```python
from build123d import *

# Parameters (mm, degrees)
F1_DEPTH = 30


with BuildPart() as f1:
    # F0 (on Front) → F1 (new body)
    with BuildSketch(Plane.XZ):
        Polygon((30, 50), (30, 0), (1135, 0), (1135, 50), (1170, 50), (1170, 150), (1135, 150), (1135, 200), (30, 200), (30, 150), (-5, 150), (-5, 50), align=None)
        with BuildLine():
            Line((312.5, 50), (112.5, 50))
            ThreePointArc((112.5, 50), (62.5, 100), (112.5, 150))
            Line((112.5, 150), (312.5, 150))
            ThreePointArc((312.5, 150), (362.5, 100), (312.5, 50))
        make_face(mode=Mode.SUBTRACT)
        with BuildLine():
            Line((682.5, 50), (482.5, 50))
            ThreePointArc((482.5, 50), (432.5, 100), (482.5, 150))
            Line((482.5, 150), (682.5, 150))
            ThreePointArc((682.5, 150), (732.5, 100), (682.5, 50))
        make_face(mode=Mode.SUBTRACT)
        with BuildLine():
            Line((1052.5, 50), (852.5, 50))
            ThreePointArc((852.5, 50), (802.5, 100), (852.5, 150))
            Line((852.5, 150), (1052.5, 150))
            ThreePointArc((1052.5, 150), (1102.5, 100), (1052.5, 50))
        make_face(mode=Mode.SUBTRACT)
    extrude(amount=F1_DEPTH)


solid = f1.part
```
The model under review builds one solid part; all positions refer to its coordinate system, in mm. A direction names the side the tool comes from. Coordinates: 2 decimals unless noted, no trailing zeros. Write each loop counter-clockwise with the first axis right and the second up, starting at its lowest first coordinate (ties: lowest second). Pieces come first, ordered by that corner, then holes. Notation, with made-up numbers: (20.5, 52) -> (51.5, 52) arc R22 ccw to (51.5, 69) -> close; hole circle Ø8 at (60.5, 86). An arc over 180 degrees is marked (long way). One line per item, written item: value. Start each with the question number.
Q1. Clearance check with flat-ended pins moving along their axes: P1, Ø9, axis at x = 1157.5, y = -20, coming from the -Z side; P2, Ø9, axis at y = -20.5, z = 168.5, coming from the -X side; P3, Ø15, axis at x = 5.5, y = -15, coming from the +Z side. State where each tip first meets the part, or that it passes through.
Q2. To check wall thickness, follow probe 1 along Z at (x, y) = (303, -5); probe 2 along X at (y, z) = (-16, 138); probe 3 along X at (y, z) = (-14, 54.5). State the ranges of each line that lie inside material, in increasing order.
Q3. The part is to be moulded in two halves that separate along X. For faces 1 (the face through (1135, -15, 175)), 2 (the face through (584, -15, 50)), 3 (the face through (-5, -15, 101)), say which applies: +X half, -X half, draft (parallel to the pull), parting line (faces both ways), or undercut.
Q4. Add section A-A, the plane x = 990. Give the boundary of the cut face in (y, z), then the cut area to 3 significant figures.
Q5. Add section C-C, the plane y = -20.75. Give the boundary of the cut face in (x, z), then the cut area to 3 significant figures.
Q6. For faces 4 (the face through (30, -15, 175)), 5 (the face through (30, -15, 25)), 6 (the face through (954, -15, 50)), list the 3-axis set-ups (+Z, -Z, +X, -X, +Y, -Y) from which the entire face can be reached by the end or side of a thin tool; tool diameter is ignored.
Q7. Add section B-B, the plane z = 100. Give the boundary of the cut face in (x, y), then the cut area to 3 significant figures.
Q8. Add section D-D, the plane z = 13. Give the boundary of the cut face in (x, y), then the cut area to 4 significant figures.
Response:
1. P1: z = 50
1. P2: x = 30
1. P3: z = 150
2. probe 1: 0 to 50, 150 to 200
2. probe 2: -5 to 80, 345 to 450, 715 to 820, 1085 to 1170
2. probe 3: -5 to 91.77, 333.23 to 461.77, 703.23 to 831.77, 1073.23 to 1170
3. face 1: +X half
3. face 2: undercut
3. face 3: -X half
4. outline: (-30, 0) -> (0, 0) -> (0, 50) -> (-30, 50) -> close; (-30, 150) -> (0, 150) -> (0, 200) -> (-30, 200) -> close
4. area: 3,000 mm²
5. outline: (-5, 50) -> (30, 50) -> (30, 0) -> (1135, 0) -> (1135, 50) -> (1170, 50) -> (1170, 150) -> (1135, 150) -> (1135, 200) -> (30, 200) -> (30, 150) -> (-5, 150) -> close; hole (112.5, 50) -> (312.5, 50) arc R50 ccw to (312.5, 150) -> (112.5, 150) arc R50 ccw to start; hole (482.5, 50) -> (682.5, 50) arc R50 ccw to (682.5, 150) -> (482.5, 150) arc R50 ccw to start; hole (852.5, 50) -> (1052.5, 50) arc R50 ccw to (1052.5, 150) -> (852.5, 150) arc R50 ccw to start
5. area: 144,000 mm²
6. face 4: +Z, -X, +Y, -Y
6. face 5: -Z, -X, +Y, -Y
6. face 6: +Y, -Y
7. outline: (-5, -30) -> (62.5, -30) -> (62.5, 0) -> (-5, 0) -> close; (362.5, -30) -> (432.5, -30) -> (432.5, 0) -> (362.5, 0) -> close; (732.5, -30) -> (802.5, -30) -> (802.5, 0) -> (732.5, 0) -> close; (1102.5, -30) -> (1170, -30) -> (1170, 0) -> (1102.5, 0) -> close
7. area: 8,250 mm²
8. outline: (30, -30) -> (1135, -30) -> (1135, 0) -> (30, 0) -> close
8. area: 33,150 mm²
